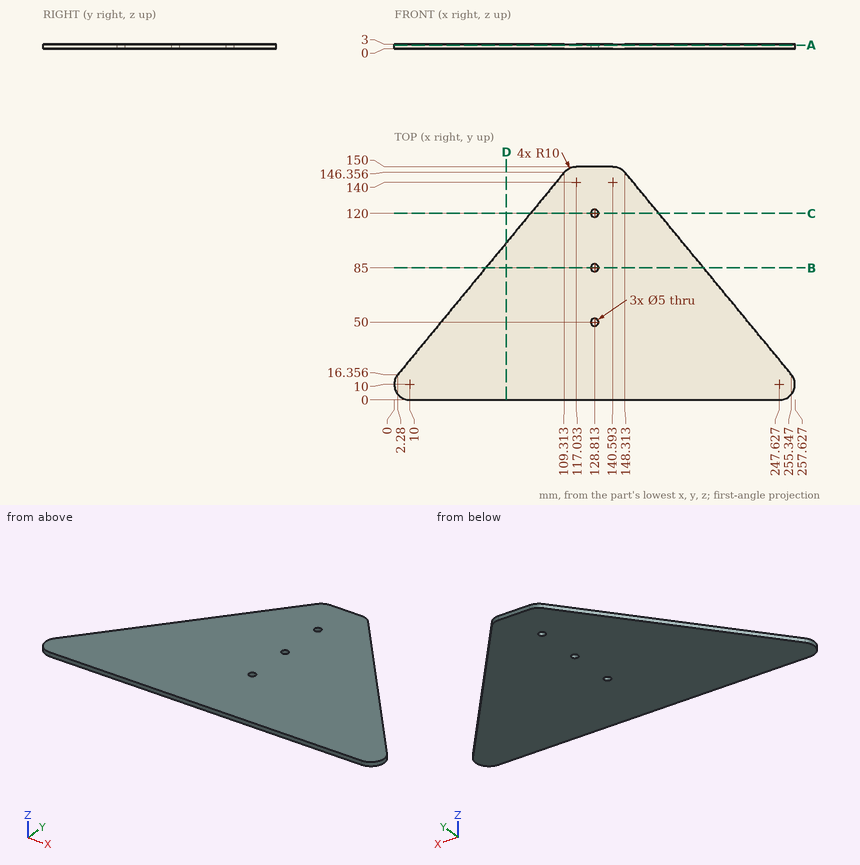
Source: three-view drawing plus pictorial views. Frame: mm from the lowest corner of the part. Round coordinates to 2 decimals unless told otherwise and drop trailing zeros. Loops run counter-clockwise (first coordinate to the right, second up) from the corner with the lowest first, then second, coordinate; pieces in that order, holes last. Notation, with made-up numbers: (52, 51) - (74, 51) arc R33 cw to (74, 83) - close; hole circle Ø9 at (49, -7.75). An arc over 180 degrees is marked (long way). Write item = value, one per line. Start each with the question number.
Item 1: Material intervals for line 1 (X direction, y = 86, z = 2.75) (1 decimal); line 2 (Y direction, x = 222.5, z = 2.35); line 3 (Y direction, x = 192.5, z = 2.3), sorted ascending.
Item 2: Section query A-A on z = 2.2. Output: boundary loops of the cut face in (x, y), plus the area to 3 significant figures.
Item 3: Section query B-B on y = 85. Output: boundary loops of the cut face in (x, z).
Item 4: First-contact query: pin 1 Ø3 at (x, y) = (128.81, 50) entering from +Z; pin 2 Ø1 at (y, z) = (133, 2.5) entering from -X (1 decimal). Flat tips, straight axial feed; report the tip coordinate or a pass-through.
Item 5: Section query D-D on x = 72. Output: boundary loops of the cut face in (y, z), plus the area to 3 significant figures.
Item 6: Section query C-C on y = 120. Output: boundary loops of the cut face in (x, z).
Results list:
q1.line_1 = 59.6 to 126.5, 131.1 to 198
q1.line_2 = 0 to 56.25
q1.line_3 = 0 to 92.69
q2.outline = (2.28, 16.36) arc R10 ccw to (10, 0) - (247.63, 0) arc R10 ccw to (255.35, 16.36) - (148.31, 146.36) arc R10 ccw to (140.59, 150) - (117.03, 150) arc R10 ccw to (109.31, 146.36) - close; hole circle Ø5 at (128.81, 50); hole circle Ø5 at (128.81, 85); hole circle Ø5 at (128.81, 120)
q2.area = 23,200 mm²
q3.outline = (58.8, 0) - (126.31, 0) - (126.31, 3) - (58.8, 3) - close; (131.31, 0) - (198.83, 0) - (198.83, 3) - (131.31, 3) - close
q4.pin_1 = through
q4.pin_2 = 97.9
q5.outline = (0, 0) - (101.04, 0) - (101.04, 3) - (0, 3) - close
q5.area = 303 mm²
q6.outline = (87.61, 0) - (126.31, 0) - (126.31, 3) - (87.61, 3) - close; (131.31, 0) - (170.01, 0) - (170.01, 3) - (131.31, 3) - close
